For this review, take the finished solid that the model builds, in its own axes (mm). Face numbers are marked on the shaded views. A direction names the side the tool comes from. Round coordinates to 2 decimals unless told otherwise and drop trailing zeros. Order: outer loops, then holes, each group sorted by start corner. A loop starts at its lowest first (then second) coordinate and runs counter-clockwise, first axis right, second up.
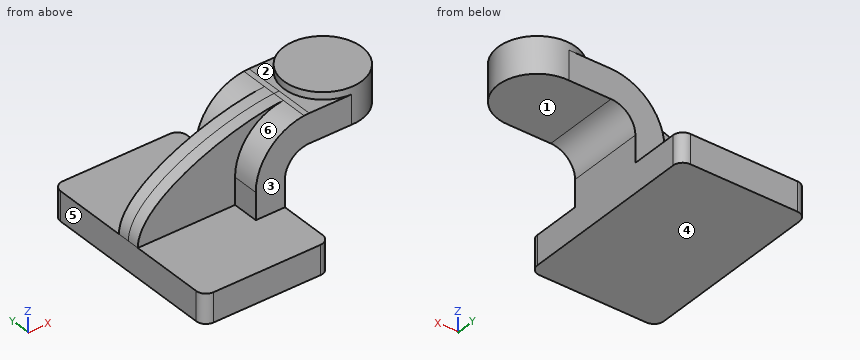
from build123d import *

# Parameters (mm, degrees)
F0_W     = 25.3809136033
F0_H     = 19.05
F1_DEPTH = 25.4
F2_DEPTH = 63.5
F3_DEPTH = 7.9375
F5_R     = 6.35


with BuildPart() as f1:
    # F0 (on Front) → F1 (new body, symmetric)
    with BuildSketch(Plane.XZ):
        with BuildLine():
            Line((22.225, 9.525), (41.275, 9.525))
            Line((41.275, 9.525), (41.275, 27.0002))
            ThreePointArc((41.275, 27.0002), (45.9246798487, 38.2255201513), (57.15, 42.8752))
            Line((57.15, 42.8752), (60.325, 42.8752))
            Line((60.325, 42.8752), (60.325, 61.9252))
            Line((60.325, 61.9252), (57.15, 61.9252))
            add(Edge.make_bspline(
                [(53.7943262834, 61.7636158119), (54.934127265, 61.8370008036), (56.0534706406, 61.8910169909), (57.15, 61.9252)],
                knots=[108.1621965606, 108.1621965606, 108.1621965606, 108.1621965606, 111.5045361635, 111.5045361635, 111.5045361635, 111.5045361635], degree=3))
            ThreePointArc((53.7943262834, 61.7636158119), (31.2950920563, 50.4795390074), (22.225, 27.0002))
            Line((22.225, 27.0002), (22.225, 9.525))
        make_face()
        with Locations((73.0154568017, 52.4002)):
            Rectangle(F0_W, F0_H)
    extrude(amount=F1_DEPTH, both=True)

    # F0 (on Front) → F2 (join, symmetric)
    with BuildSketch(Plane.XZ):
        Polygon((-41.275, 9.525), (-41.275, -9.525), (41.275, -9.525), (41.275, 9.525), (22.225, 9.525), align=None)
    extrude(amount=F2_DEPTH, both=True)

    # F0 (on Front) → F3 (join, symmetric)
    with BuildSketch(Plane.XZ):
        with BuildLine():
            add(Edge.make_bspline(
                [(-41.275, 9.525), (-41.4005826971, 36.730003512), (16.9089727739, 59.3887877429), (53.7943262834, 61.7636158119)],
                knots=[0, 0, 0, 0, 108.1621965606, 108.1621965606, 108.1621965606, 108.1621965606], degree=3))
            Line((-41.275, 9.525), (22.225, 9.525))
            Line((22.225, 9.525), (22.225, 27.0002))
            ThreePointArc((22.225, 27.0002), (31.2950920563, 50.4795390074), (53.7943262834, 61.7636158119))
        make_face()
    extrude(amount=F3_DEPTH, both=True)

    # F0 (on Front) → F4 (revolve)
    with BuildSketch(Plane.XZ):
        Polygon((85.7059136033, 66.675), (85.7059136033, 61.9252), (85.7059136033, 42.8752), (111.125, 42.8752), (111.125, 66.675), align=None)
    revolve(axis=Axis((85.7059136033, 0, 54.7751), (0, 0, 1)))

    # F5
    f5_edges = [f1.edges().sort_by_distance(p)[0] for p in [
        (41.275, -63.5, 0),
        (-41.275, -63.5, 0),
        (41.275, 63.5, 0),
        (-41.275, 63.5, 0),
    ]]
    fillet(f5_edges, radius=F5_R)


solid = f1.part
(1) Tool access review of the marked faces 1, 2 and 3: name each direction out of +Z, -Z, +X, -X, +Y, -Y from which nothing blocks a thin tool from reaching the whole face with its end or side.
(2) Add section B-B on y = 42.5. Give the boundary of the cut face in (x, z) (3 decimals).
(3) Draft analysis for pull direction Z (two halves, no side actions). For the marked faces 4, 5 and 6, state which applies: pulls with the +Z half, pulls with the -Z half, needs draft (parallel to the pull), parting line crosses it, or undercut.
(4) Clearance check with flat-ended pins moving along their axes: P1, Ø12, axis at y = -41.5, z = 3.5, coming from the +X side (3 decimals); P2, Ø2, axis at x = 61, y = 1.5, coming from the -Z side; P3, Ø2, axis at x = 37.5, z = 32, coming from the -Y side. State where each tip first meets the part, or that it passes through.
(5) Wall thickness on L1, parallel to Z at x = -34.5, y = -32.5 (3 decimals); L2, parallel to X at y = 12.5, z = 19.5 (3 decimals); L3, parallel to Y at x = 23, z = 33.5: over which ranges is each line inside the solid? List them lowest first.
(6) Add section A-A on z = 7. Give the boundary of the cut face in (x, y) (3 decimals), plus the area to 3 significant figures.
Here are the results:
1. face 1: -Z, +X, +Y, -Y
1. face 2: +Z, -X
1. face 3: +Z, +X, -X, -Y
2. outline: (-41.275, -9.525) - (41.275, -9.525) - (41.275, 9.525) - (-41.275, 9.525) - close
3. face 4: pulls with the -Z half
3. face 5: needs draft
3. face 6: pulls with the +Z half
4. P1: stops at x = 41.275
4. P2: stops at z = 42.88
4. P3: stops at y = -25.4
5. L1: z = -9.525 to 9.525
5. L2: x = 22.225 to 41.275
5. L3: y = -25.4 to 25.4
6. outline: (-41.275, -57.15) arc R6.35 ccw to (-34.925, -63.5) - (34.925, -63.5) arc R6.35 ccw to (41.275, -57.15) - (41.275, 57.15) arc R6.35 ccw to (34.925, 63.5) - (-34.925, 63.5) arc R6.35 ccw to (-41.275, 57.15) - close
6. area: 10,400 mm2
